Geometry check sheet. Reference: the model listing, model coordinates, mm. Face numbers are marked on the shaded views. A direction names the side the tool comes from. Coordinates: 2 decimals unless noted, no trailing zeros. Write each loop counter-clockwise with the first axis right and the second up, starting at its lowest first coordinate (ties: lowest second). Pieces come first, ordered by that corner, then holes.
from build123d import *

# Parameters (mm, degrees)
F0_R     = 15
F1_DEPTH = 150
F2_W     = 20
F2_H     = 20
F3_DEPTH = 15.001
F4_DEPTH = 15.001


with BuildPart() as f1:
    # F0 (on Top) → F1 (new body)
    with BuildSketch(Plane.XY):
        Circle(F0_R)
    extrude(amount=F1_DEPTH)

    # F2 (on Front) → F3 (cut, through all)
    with BuildSketch(Plane.XZ):
        with Locations((1.2132771455, 120)):
            Rectangle(F2_W, F2_H)
    extrude(amount=-F3_DEPTH, mode=Mode.SUBTRACT)

    # F2 (on Front) → F4 (cut, through all)
    with BuildSketch(Plane.XZ):
        with Locations((1.2132771455, 120)):
            Rectangle(F2_W, F2_H)
    extrude(amount=F4_DEPTH, mode=Mode.SUBTRACT)


solid = f1.part
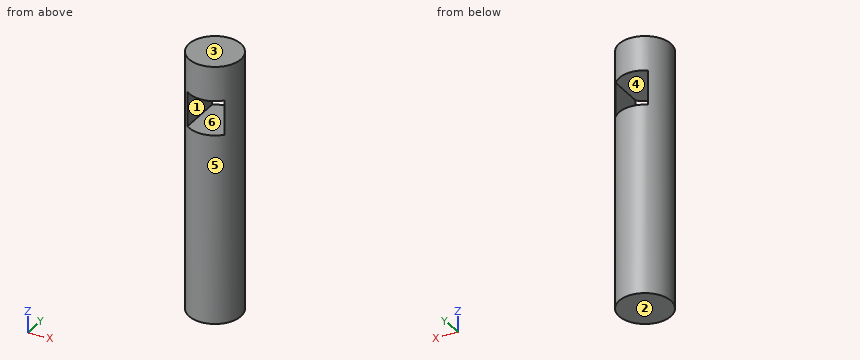
1. Thickness scan on line 1 along Z through (x, y) = (-0.5, 10); line 2 along X through (y, z) = (0.5, 127); line 3 along X through (y, z) = (-0.75, 142). Record the ranges inside material, lowest first.
Computed values:
line 1: z = 0 to 110, 130 to 150
line 2: x = -14.99 to -8.79, 11.21 to 14.99
line 3: x = -14.98 to 14.98
2. Sectioned sample at B-B, the plane y = 0. Record the boundary of the cut face in (x, z).
Computed values:
outline: (-15, 0) - (15, 0) - (15, 150) - (-15, 150) - close; hole (-8.79, 110) - (11.21, 110) - (11.21, 130) - (-8.79, 130) - close
3. Access from +Z, -Z, +X, -X, +Y, -Y to the whole of each face (thin tool, end or side, straight path). Record for the marked faces 1 and 2.
Computed values:
face 1: +Y, -Y
face 2: -Z, +X, -X, +Y, -Y
4. Gauge pin test, flat ends, axial feed: pin 1 Ø6 at (x, z) = (5.5, 84) entering from -Y; pin 2 Ø6 at (y, z) = (-3.5, 116.5) entering from -X; pin 3 Ø6 at (x, z) = (-3.5, 42.5) entering from +Y; pin 4 Ø10 at (x, y) = (-3.5, -6) entering from -Z. Record the tip position at first contact, or that the pin passes through.
Computed values:
pin 1: stops at y = -14.79
pin 2: stops at x = -14.99
pin 3: stops at y = 14.99
pin 4: stops at z = 0
5. Sectioned sample at C-C, the plane z = 114.5. Record the boundary of the cut face in (x, y), and give its area (3 significant figures).
Computed values:
outline: (-8.79, -12.16) - (-8.79, 12.16) arc R15 ccw to start; (11.21, -9.96) arc R15 ccw to (11.21, 9.96) - close
area: 158 mm2
6. Sectioned sample at A-A, the plane x = 0. Record the boundary of the cut face in (y, z).
Computed values:
outline: (-15, 0) - (15, 0) - (15, 110) - (-15, 110) - close; (-15, 130) - (15, 130) - (15, 150) - (-15, 150) - close
7. Draft check along X on the marked faces 3, 4, 5 and 6. Enter one of: released by +X, released by -X, zero draft, split by the parting line, or undercut.
Computed values:
face 3: zero draft
face 4: undercut
face 5: split by the parting line
face 6: undercut
8. Sectioned sample at D-D, the plane z = 40.5. Record the boundary of the cut face in (x, y).
Computed values:
outline: circle Ø30 at (0, 0)
